```python
from build123d import *

# Parameters (mm, degrees)
SKETCH1_R           = 2.5
BOSS_EXTRUDE1_DEPTH = 8
BOSS_EXTRUDE2_START = -5
SKETCH2_R           = 2.5
BOSS_EXTRUDE2_DEPTH = 5
SKETCH3_OUTSIDE_W   = 135.206
SKETCH3_OUTSIDE_H   = 97.706
CUT_EXTRUDE2_DEPTH  = 3


with BuildPart() as part:
    # Sketch1 → Boss-Extrude1 (new body)
    with BuildSketch(Plane(origin=(0, 0, 0), x_dir=(1, 0, 0), z_dir=(0, 1, 0))):
        with BuildLine():
            Line((0, 10), (87.5, 10))
            ThreePointArc((87.5, 10), (97.5, 0), (87.5, -10))
            Line((87.5, -10), (0, -10))
            ThreePointArc((0, -10), (-10, 0), (0, 10))
        make_face()
        with Locations(Location((0, 0, 0), (0, 0, 270))):
            Circle(SKETCH1_R, mode=Mode.SUBTRACT)
        with BuildLine():
            Line((87.5, -4), (82.5, -4))
            ThreePointArc((82.5, -4), (78.5, 0), (82.5, 4))
            Line((82.5, 4), (87.5, 4))
            ThreePointArc((87.5, 4), (91.5, 0), (87.5, -4))
        make_face(mode=Mode.SUBTRACT)
    extrude(amount=BOSS_EXTRUDE1_DEPTH)

    # Sketch2 → Boss-Extrude2 (add)
    with BuildSketch(Plane(origin=(0, 8, 0), x_dir=(1, 0, 0), z_dir=(0, 1, 0)).offset(BOSS_EXTRUDE2_START)):
        with BuildLine():
            Line((-10, 0), (-10, 50))
            ThreePointArc((-10, 50), (0, 60), (10, 50))
            Line((10, 50), (10, 0))
            ThreePointArc((10, 0), (0, -10), (-10, 0))
        make_face()
        with Locations(Location((0, 0, 0), (0, 0, 270))):
            Circle(SKETCH2_R, mode=Mode.SUBTRACT)
        with Locations(Location((0, 50, 0), (0, 0, 270))):
            Circle(SKETCH2_R, mode=Mode.SUBTRACT)
    extrude(amount=BOSS_EXTRUDE2_DEPTH)

    # Sketch3 outside → Cut-Extrude2 (cut)
    with BuildSketch(Plane.XZ):
        with Locations((43.75, -25)):
            Rectangle(SKETCH3_OUTSIDE_W, SKETCH3_OUTSIDE_H)
        with BuildLine():
            Line((87.5, -10), (77.5, -10))
            ThreePointArc((77.5, -10), (67.5, 0), (77.5, 10))
            Line((77.5, 10), (87.5, 10))
            ThreePointArc((87.5, 10), (97.5, 0), (87.5, -10))
        make_face(mode=Mode.SUBTRACT)
    extrude(amount=-CUT_EXTRUDE2_DEPTH, mode=Mode.SUBTRACT)


solid = part.part
```
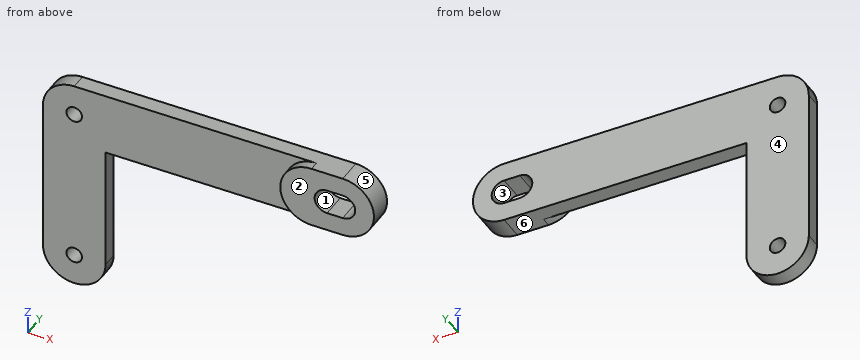
The listing builds one solid part. Answer for the finished solid, in the listing's coordinates (mm). Face numbers are marked on the shaded views. A direction names the side the tool comes from. Give positions to 0.01 mm unless a question says otherwise; leave off trailing zeros. Write each loop counter-clockwise with the first axis right and the second up, starting at its lowest first coordinate (ties: lowest second). Pieces come first, ordered by that corner, then holes. Notation, with made-up numbers: (65, 88) -> (114, 88) arc R24 ccw to (114, 115) -> close; hole circle Ø7 at (-22.5, 43.25). An arc over 180 degrees is marked (long way). Write item = value, one per line. Start each with the question number.
1) Determine the mould class of the marked faces 3, 4, 5 and 6 for opening direction Z: +Z half, -Z half, draft (parallel to the pull), parting line (faces both ways), or undercut.
2) The part is cut by section C-C, the plane z = -26.5. Determine the outline of the cut face in (x, y), and give its area (3 significant figures).
3) The part is cut by section A-A, the plane y = 1.5. Determine the outline of the cut face in (x, z).
4) The part is cut by section B-B, the plane x = 33.5. Determine the outline of the cut face in (y, z).
5) Straight lines are drawn through the part: line 1 along X through (y, z) = (4.5, -50); line 2 along X through (y, z) = (7.25, -15); line 3 along Y through (x, z) = (9, -6). For each, find the intervals that lie inside material, in ascending order.
6) Which of the six approach directions +Z, -Z, +X, -X, +Y, -Y give full straight-line access (tool end or side, diameter ignored) to the marked faces 1 and 2?
7) Each of these flat-tipped pins is pushed along its axis until it touches: pin 1 (6.5 mm diameter, centred on x = 0, z = -50, fed in from +Y); pin 2 (1 mm diameter, centred on x = 57.5, y = 5, fed in from -Z); pin 3 (1.5 mm diameter, centred on y = 6, z = -31.5, fed in from +X). Where does it stop, or does it pass through?
Solutions:
q1.face_3 = undercut
q1.face_4 = draft
q1.face_5 = parting line
q1.face_6 = -Z half
q2.outline = (-10, 3) -> (10, 3) -> (10, 8) -> (-10, 8) -> close
q2.area = 100 mm²
q3.outline = (77.5, -10) -> (87.5, -10) arc R10 ccw to (87.5, 10) -> (77.5, 10) arc R10 ccw to start; hole (82.5, -4) -> (87.5, -4) arc R4 ccw to (87.5, 4) -> (82.5, 4) arc R4 ccw to start
q4.outline = (3, -10) -> (8, -10) -> (8, 10) -> (3, 10) -> close
q5.line_1 = -10 to -2.5, 2.5 to 10
q5.line_2 = -10 to 10
q5.line_3 = 3 to 8
q6.face_1 = +Y, -Y
q6.face_2 = +Z, -Z, +X, -X, -Y
q7.pin_1 = 8
q7.pin_2 = -10
q7.pin_3 = 10
